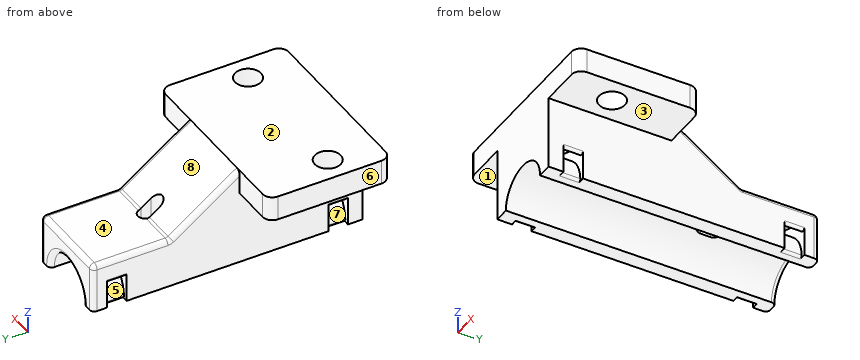
from build123d import *

# Parameters (mm, degrees)
BOSS_EXTRUDE1_DEPTH  = 20
M5_CLEARANCE_HOLE1_D = 5.3
SKETCH11_W           = 1.8
SKETCH11_H           = 4
FILLET2_START        = 3
FILLET2_DEPTH        = 4
MOVE_FACE1_BY        = 5
BOSS_EXTRUDE2_DEPTH  = 30
FILLET1_R            = 2
SKETCH13_W           = 10
SKETCH13_H           = 30
CUT_EXTRUDE1_DEPTH   = 65.876806449
CHAMFER3_SIZE        = 14.281480067
CHAMFER3_SIZE_2      = 10
FILLET3_R            = 1
CUT_EXTRUDE2_DEPTH   = 62.530480341


with BuildPart() as part:
    # Sketch4 → Boss-Extrude1 (new body)
    with BuildSketch(Plane(origin=(0, 0, 0), x_dir=(1, 0, 0), z_dir=(0, 1, 0))):
        with BuildLine():
            Line((19, 0), (-19, 0))
            Line((-19, 0), (-19, 5))
            Line((-19, 5), (-9, 5))
            Line((-9, 5), (-9, 20))
            Line((-9, 20), (-6, 20))
            ThreePointArc((-6, 20), (0, 14), (6, 20))
            Line((6, 20), (9, 20))
            Line((9, 20), (9, 5))
            Line((9, 5), (19, 5))
            Line((19, 5), (19, 0))
        make_face()
    extrude(amount=BOSS_EXTRUDE1_DEPTH)

    # M5 Clearance Hole1 (through all)
    with Locations(Plane(origin=(0, 0, -5), x_dir=(-1, 0, 0), z_dir=(0, 0, -1))):
        with Locations((-14, 10), (14, 10)):
            Hole(M5_CLEARANCE_HOLE1_D / 2)

    # Cut-Sweep1: sweep along a path in Sketch10
    with BuildLine(Plane(origin=(0, 5, 0), x_dir=(1, 0, 0), z_dir=(0, 1, 0))) as cut_sweep1_path:
        CenterArc((0, 20), 6, 0, 360)
    # Sketch11 → Cut-Sweep1 (sweep, cut)
    with BuildSketch(Plane(origin=(0, 0, -20), x_dir=(-1, 0, 0), z_dir=(0, 0, -1))):
        with Locations((-9, 5)):
            Rectangle(SKETCH11_W, SKETCH11_H)
    cut_sweep1 = sweep(path=cut_sweep1_path.line, mode=Mode.SUBTRACT)

    # Fillet2: read off the stored shape, not the designer's step
    # Fillet2 outline → Fillet2 (cut)
    with BuildSketch(Plane(origin=(0, 0, 0), x_dir=(1, 0, 0), z_dir=(0, 1, 0)).offset(FILLET2_START)):
        with BuildLine():
            ThreePointArc((7.583534796, 20), (7.948532993, 19.841725498), (8.082451559, 19.467105263))
            ThreePointArc((8.082451559, 19.467105263), (8.095611701, 19.733408201), (8.1, 20))
            Line((8.1, 20), (7.583534796, 20))
        make_face()
        with BuildLine():
            ThreePointArc((-8.1, 20), (-8.095611701, 19.733408201), (-8.082451559, 19.467105263))
            ThreePointArc((-8.082451559, 19.467105263), (-7.948532993, 19.841725498), (-7.583534796, 20))
            Line((-7.583534796, 20), (-8.1, 20))
        make_face()
        with BuildLine():
            Line((9, 14.007504693), (9, 15.875681875))
            ThreePointArc((9, 15.875681875), (8.582114467, 15.064687318), (8.091346154, 14.295605429))
            ThreePointArc((8.091346154, 14.295605429), (8.651117631, 14.484121375), (9, 14.007504693))
        make_face()
        with BuildLine():
            ThreePointArc((-8.091346154, 14.295605429), (-8.582114467, 15.064687318), (-9, 15.875681875))
            Line((-9, 15.875681875), (-9, 14.007504693))
            ThreePointArc((-9, 14.007504693), (-8.651117631, 14.484121375), (-8.091346154, 14.295605429))
        make_face()
    fillet2 = extrude(amount=FILLET2_DEPTH, mode=Mode.SUBTRACT)

    # Move Face1: a face moved outward by 5.0
    extrude(part.faces().sort_by_distance((0, 20, -7.09633707))[0], amount=MOVE_FACE1_BY, dir=(0, 1, 0))

    # Sketch12 → Boss-Extrude2 (add)
    with BuildSketch(Plane(origin=(0, 25, 0), x_dir=(1, 0, 0), z_dir=(0, 1, 0))):
        with BuildLine():
            Line((-9, 5), (-9, 0))
            Line((-9, 0), (9, 0))
            Line((9, 0), (9, 5))
            Line((9, 5), (9, 20))
            Line((9, 20), (6, 20))
            ThreePointArc((6, 20), (0, 14), (-6, 20))
            Line((-6, 20), (-9, 20))
            Line((-9, 20), (-9, 5))
        make_face()
    extrude(amount=BOSS_EXTRUDE2_DEPTH)

    # Fillet1
    fillet1_edges = [part.edges().sort_by_distance(p)[0] for p in [
        (19, 25, -2.5),
        (19, 0, -2.5),
        (-19, 0, -2.5),
        (-19, 25, -2.5),
    ]]
    fillet(fillet1_edges, radius=FILLET1_R)

    # Sketch13 → Cut-Extrude1 (cut, through all)
    with BuildSketch(Plane.ZY.offset(9)):
        with Locations((-5, 40)):
            Rectangle(SKETCH13_W, SKETCH13_H)
    extrude(amount=-CUT_EXTRUDE1_DEPTH, mode=Mode.SUBTRACT)

    # Chamfer3
    # the kernel refuses this chamfer: 14.281480067, 10 mm, written as the material it adds along each edge
    with BuildSketch(Plane(origin=(-9, 25, -10), x_dir=(0, 1, 0), z_dir=(1, 0, 0))) as chamfer3_piece_1_section:
        Polygon((CHAMFER3_SIZE, 0), (0, CHAMFER3_SIZE_2), (0, 0), align=None)
    chamfer3_piece_1 = extrude(amount=18, mode=Mode.PRIVATE)
    chamfer3_piece_1 = split(chamfer3_piece_1, bisect_by=Plane(origin=(-9, 25, 0), z_dir=(0, 0, -1)), keep=Keep.TOP, mode=Mode.PRIVATE)
    add(chamfer3_piece_1)

    # Fillet3
    fillet3_edges = [part.edges().sort_by_distance(p)[0] for p in [
        (0, 55, -14),
        (-9, 55, -15),
        (9, 55, -15),
        (0, 55, -10),
        (9, 47.140740034, -10),
        (-9, 47.140740034, -10),
        (0, 39.281480067, -10),
        (-9, 32.140740034, -5),
        (9, 32.140740034, -5),
    ]]
    fillet(fillet3_edges, radius=FILLET3_R)

    # Mirror1: Cut-Sweep1, Fillet2 across plane
    add(cut_sweep1.mirror(Plane.ZX.offset(27.5)), mode=Mode.SUBTRACT)
    add(fillet2.mirror(Plane.ZX.offset(27.5)), mode=Mode.SUBTRACT)

    # Sketch14 → Cut-Extrude2 (cut, through all)
    with BuildSketch(Plane(origin=(0, 0, -20), x_dir=(-1, 0, 0), z_dir=(0, 0, -1))):
        with BuildLine():
            Line((-1.5, 37), (-1.5, 39))
            ThreePointArc((-1.5, 39), (0, 40.5), (1.5, 39))
            Line((1.5, 39), (1.5, 37))
            ThreePointArc((1.5, 37), (0, 35.5), (-1.5, 37))
        make_face()
    extrude(amount=-CUT_EXTRUDE2_DEPTH, mode=Mode.SUBTRACT)


solid = part.part
Geometry: final body of the model. Coordinates: model frame, mm. Face numbers are marked on the shaded views. A direction names the side the tool comes from. Round coordinates to 2 decimals unless told otherwise and drop trailing zeros. Order: outer loops, then holes, each group sorted by start corner. A loop starts at its lowest first (then second) coordinate and runs counter-clockwise, first axis right, second up. Notation, with made-up numbers: (46, 64) - (88, 64) arc R4 cw to (88, 71) - close; hole circle Ø5 at (-29.75, -21.5). An arc over 180 degrees is marked (long way). Write each question's results on one line, items separated by ' | '.
Item 1: Section C-C, the plane y = 50. Return the cut outline in (x, z).
Completed:
outline: (-9, -14.01) arc R0.5 ccw to (-8.09, -14.3) arc R9.9 cw to (8.09, -14.3) arc R0.5 ccw to (9, -14.01) - (9, -11) arc R1 ccw to (8, -10) - (-8, -10) arc R1 ccw to (-9, -11) - close; (-8.08, -19.47) arc R0.5 ccw to (-7.58, -20) - (-6, -20) arc R6 cw to (6, -20) - (7.58, -20) arc R0.5 ccw to (8.08, -19.47) arc R8.1 ccw to start
Item 2: First-contact query: pin 1 Ø5 at (y, z) = (25, -7) entering from +X; pin 2 Ø8 at (x, z) = (0.5, -17.5) entering from +Y; pin 3 Ø5 at (x, z) = (13, -16) entering from -Y; pin 4 Ø1.5 at (x, z) = (11, -3) entering from +Y. Flat tips, straight axial feed; report the tip coordinate or a pass-through.
Completed:
pin 1: x = 18.94 | pin 2: y = 54.89 | pin 3: through | pin 4: y = 25
Item 3: Section B-B, the plane x = -14. Return the cut outline in (y, z), and give its area (3 significant figures).
Completed:
outline: (0, -5) - (7.35, -5) - (7.35, 0) - (0, 0) - close; (12.65, -5) - (25, -5) - (25, 0) - (12.65, 0) - close | area: 98.5 mm^2
Item 4: Section A-A, the plane y = 10. Return the cut outline in (x, z).
Completed:
outline: (-19, -5) - (-16.65, -5) - (-16.65, 0) - (-19, 0) - close; (-11.35, -5) - (-9, -5) - (-9, -20) - (-6, -20) arc R6 cw to (6, -20) - (9, -20) - (9, -5) - (11.35, -5) - (11.35, 0) - (-11.35, 0) - close; (16.65, -5) - (19, -5) - (19, 0) - (16.65, 0) - close
Item 5: Reachability of the marked faces 1, 2, 3 and 4 from +Z, -Z, +X, -X, +Y, -Y: full face, straight path, thin tool, end or side. Return the list, or none.
Completed:
face 1: -Z, -X, +Y, -Y | face 2: +Z, +X, -X, +Y, -Y | face 3: -Z, +X, +Y, -Y | face 4: +Z, +X, -X, +Y
Item 6: Section D-D, the plane y = 19. Return the cut outline in (x, z).
Completed:
outline: (-19, -5) - (-9, -5) - (-9, -20) - (-6, -20) arc R6 cw to (6, -20) - (9, -20) - (9, -5) - (19, -5) - (19, 0) - (-19, 0) - close
Item 7: Mould query, pull axis Z, two halves, no side actions, for the marked faces 5, 6, 7 and 8. Classes: pulls with the +Z half, pulls with the -Z half, needs draft (parallel to the pull), parting line crosses it, or undercut.
Completed:
face 5: undercut | face 6: needs draft | face 7: undercut | face 8: pulls with the +Z half
Item 8: Material intervals for line 1 along Y through (x, z) = (-8, -18); line 2 along Y through (x, z) = (14, -3.55); line 3 along Z through (x, y) = (0.5, 9), sorted ascending. Write a range as [from, to].
Completed:
line 1: [0, 3], [7, 48], [52, 55] | line 2: [0, 7.35], [12.65, 25] | line 3: [-14.02, 0]
